Geometry: final body of the model. Coordinates: model frame, mm. Face numbers are marked on the shaded views. Give positions to 0.01 mm unless a question says otherwise; leave off trailing zeros. Write each loop counter-clockwise with the first axis right and the second up, starting at its lowest first coordinate (ties: lowest second). Pieces come first, ordered by that corner, then holes. Notation, with made-up numbers: (-29, 85) - (-16, 85) arc R34 ccw to (-16, 122) - close; hole circle Ø10 at (-14.75, -16). An arc over 180 degrees is marked (long way). Return JSON: item names as keys, results as strings.
from build123d import *

# Parameters (mm, degrees)
SALIENTE_EXTRUIR1_DEPTH = 38.8


with BuildPart() as part:
    # Croquis1 → Saliente-Extruir1 (new body)
    with BuildSketch(Plane.XY):
        with BuildLine():
            Line((620.448376311, 354.810426019), (619.409039206, 356.610610691))
            Line((619.409039206, 356.610610691), (617.330364997, 356.610610691))
            ThreePointArc((617.330364997, 356.610610691), (616.536614955, 355.235795338), (614.949114914, 355.23579541))
            ThreePointArc((614.949114914, 355.23579541), (614.368049644, 355.816860732), (614.155364997, 356.610610691))
            Line((614.155364997, 356.610610691), (612.076690788, 356.610610691))
            Line((612.076690788, 356.610610691), (611.037353683, 354.810426019))
            ThreePointArc((611.037353683, 354.810426019), (611.618419011, 352.641860691), (609.449853683, 352.060795362))
            Line((609.449853683, 352.060795362), (608.410516578, 350.260610691))
            Line((608.410516578, 350.260610691), (609.449853683, 348.460426019))
            ThreePointArc((609.449853683, 348.460426019), (611.618419011, 347.879360691), (611.037353683, 345.710795362))
            Line((611.037353683, 345.710795362), (612.076690788, 343.910610691))
            Line((612.076690788, 343.910610691), (614.155364997, 343.910610691))
            ThreePointArc((614.155364997, 343.910610691), (615.742864997, 345.498110691), (617.330364997, 343.910610691))
            Line((617.330364997, 343.910610691), (619.409039206, 343.910610691))
            Line((619.409039206, 343.910610691), (620.448376311, 345.710795362))
            ThreePointArc((620.448376311, 345.710795362), (619.867310982, 347.879360691), (622.035876311, 348.460426019))
            Line((622.035876311, 348.460426019), (623.075213416, 350.260610691))
            Line((623.075213416, 350.260610691), (622.035876311, 352.060795362))
            ThreePointArc((622.035876311, 352.060795362), (621.242126263, 351.848110691), (620.448376228, 352.06079541))
            ThreePointArc((620.448376228, 352.06079541), (619.654626311, 353.435610739), (620.448376311, 354.810426019))
        make_face()
        with BuildLine():
            ThreePointArc((614.276014843, 347.719952052), (618.283523635, 348.793760537), (617.209715151, 352.801269329))
            ThreePointArc((617.209715151, 352.801269329), (613.202206359, 351.727460845), (614.276014843, 347.719952052))
        make_face(mode=Mode.SUBTRACT)
    extrude(amount=-SALIENTE_EXTRUIR1_DEPTH)


solid = part.part
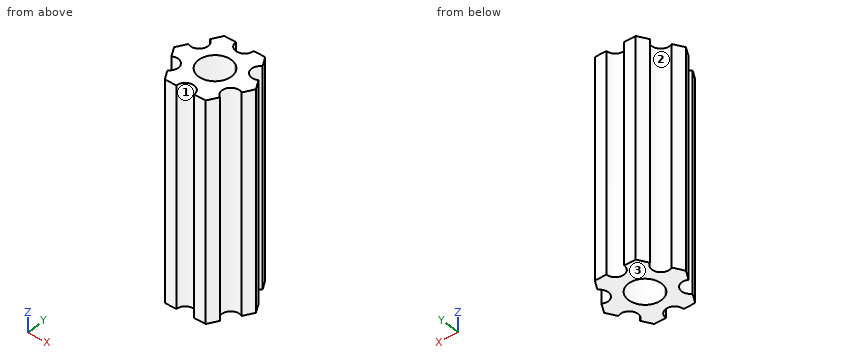
Q1. Mould query, pull axis X, two halves, no side actions, for the marked faces 1, 2 and 3. Classes: pulls with the +X half, pulls with the -X half, needs draft (parallel to the pull), parting line crosses it, or undercut.
Answer key:
{"face 1": "undercut", "face 2": "undercut", "face 3": "needs draft"}
Q2. Section query D-D, the plane x = 621. Return the cut outline in (y, z).
Answer key:
{"outline": "(348.65, -38.8) - (351.87, -38.8) - (351.87, 0) - (348.65, 0) - close"}
Q3. Section query A-A, the plane z = -27. Return the cut outline in (x, y) (1 decimal), plus the area to 3 significant figures.
Answer key:
{"outline": "(608.4, 350.3) - (609.4, 348.5) arc R1.6 cw to (611, 345.7) - (612.1, 343.9) - (614.2, 343.9) arc R1.6 cw to (617.3, 343.9) - (619.4, 343.9) - (620.4, 345.7) arc R1.6 cw to (622, 348.5) - (623.1, 350.3) - (622, 352.1) arc R1.6 cw to (620.4, 354.8) - (619.4, 356.6) - (617.3, 356.6) arc R1.6 cw to (614.2, 356.6) - (612.1, 356.6) - (611, 354.8) arc R1.6 cw to (609.4, 352.1) - close; hole circle Ø5.9 at (615.7, 350.3)", "area": "88.9 mm^2"}
Q4. Pin query (flat end, axial travel): P1, Ø4, axis at y = 352.5, z = -33.5, coming from the -X side; P2, Ø1, axis at x = 617, y = 351.5, coming from the -Z side; P3, Ø6, axis at y = 348, z = -30.5, coming from the -X side; P4, Ø1.5, axis at x = 616.5, y = 354.5, coming from the +Z side. Return the tip coordinate at first contact, or that it passes through.
Answer key:
{"P1": "stops at x = 608.55", "P2": "passes through", "P3": "stops at x = 608.41", "P4": "stops at z = 0"}
Q5. Section query B-B, the plane x = 618. Return the cut outline in (y, z).
Answer key:
{"outline": "(343.91, -38.8) - (348.39, -38.8) - (348.39, 0) - (343.91, 0) - close; (352.13, -38.8) - (356.61, -38.8) - (356.61, 0) - (352.13, 0) - close"}
Q6. Material intervals for probe 1 along X at (y, z) = (350.25, -36.5); probe 2 along Y at (x, z) = (620, -29); probe 3 along Y at (x, z) = (620.25, -2.5), sorted ascending. Write a range as [from, to].
Answer key:
{"probe 1": "x = [608.42, 612.81], [618.68, 623.07]", "probe 2": "y = [344.93, 346.1], [348.07, 352.45], [354.42, 355.59]", "probe 3": "y = [345.37, 345.85], [348.32, 352.2], [354.67, 355.15]"}
Q7. Section query C-C, the plane x = 613.5. Return the cut outline in (y, z).
Answer key:
{"outline": "(343.91, -38.8) - (348.37, -38.8) - (348.37, 0) - (343.91, 0) - close; (352.15, -38.8) - (356.61, -38.8) - (356.61, 0) - (352.15, 0) - close"}
